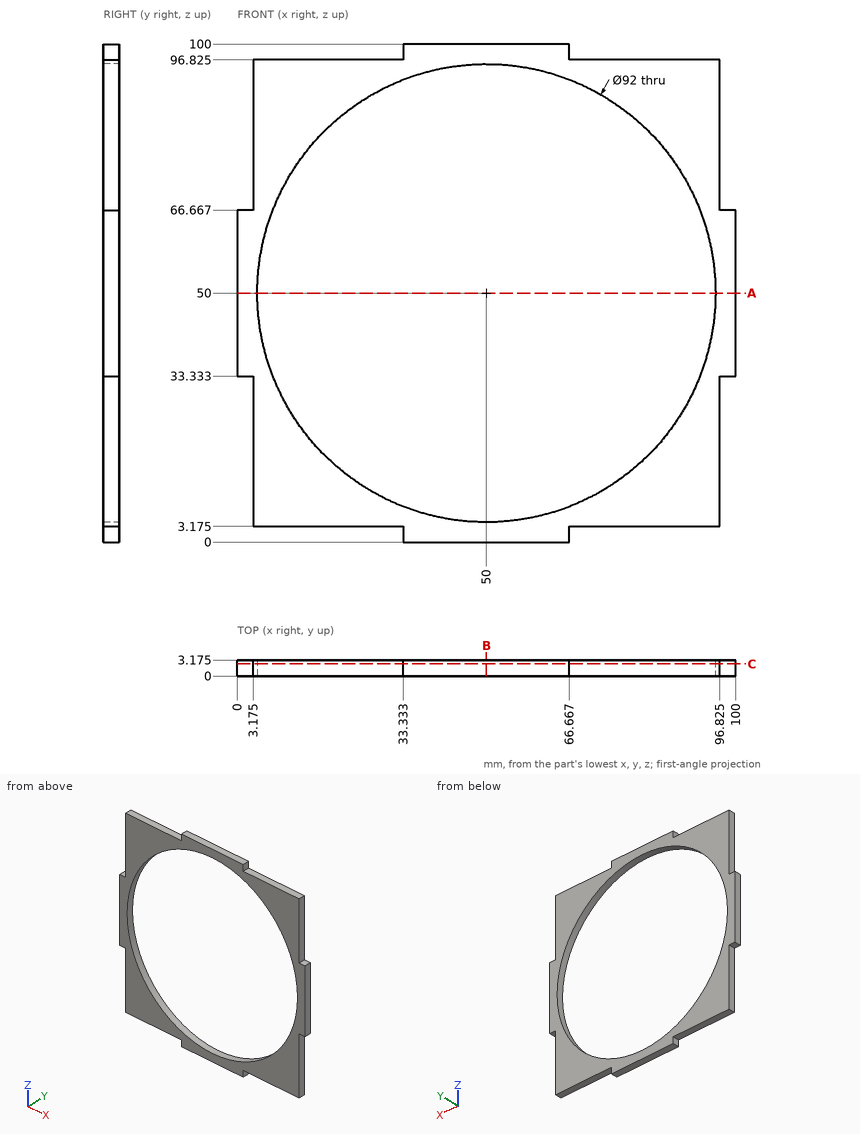
Geometry check sheet. Reference: drawing and pictorial views, mm from the part's lowest x, y, z. Round coordinates to 2 decimals unless told otherwise and drop trailing zeros. Loops run counter-clockwise (first coordinate to the right, second up) from the corner with the lowest first, then second, coordinate; pieces in that order, holes last. Notation, with made-up numbers: M 51,6 L 72,6 A14 cw 72,10 Z; hole C -36,46 d6. An arc over 180 degrees is marked long. Return JSON: item names as keys, results as strings. Group by question number.
(1) Go/stop test with flat-tipped pins: pin 1 (1 mm diameter, centred on y = 1.5, z = 1, fed in from -X); pin 2 (1 mm diameter, centred on y = 1, z = 2, fed in from +X); pin 3 (1 mm diameter, centred on y = 2, z = 21, fed in from -X) (3 decimals). Record where each tip stops, or that it passes through.
(2) Section check A-A, the plane z = 50. Enter the section's corners in (x, y) (1 decimal), and give its area (3 significant figures).
(3) Section check C-C, the plane y = 2.45. Enter the section's corners in (x, z) (1 decimal).
(4) Section check B-B, the plane x = 50. Enter the section's corners in (y, z) (1 decimal), and give its area (3 significant figures).
(5) Scan lines: line 1 along X through (y, z) = (1.9, 50); line 2 along Z through (x, y) = (76.5, 3) (1 decimal). Record each from-to range of solid material in increasing order. Write a range as [from, to].
Data:
{
 "1": {"pin 1": "x = 33.33", "pin 2": "x = 66.67", "pin 3": "x = 3.175"},
 "2": {"outline": "M 0,0 L 4,0 L 4,3.2 L 0,3.2 Z; M 96,0 L 100,0 L 100,3.2 L 96,3.2 Z", "area": "25.4 mm²"},
 "3": {"outline": "M 0,33.3 L 3.2,33.3 L 3.2,3.2 L 33.3,3.2 L 33.3,0 L 66.7,0 L 66.7,3.2 L 96.8,3.2 L 96.8,33.3 L 100,33.3 L 100,66.7 L 96.8,66.7 L 96.8,96.8 L 66.7,96.8 L 66.7,100 L 33.3,100 L 33.3,96.8 L 3.2,96.8 L 3.2,66.7 L 0,66.7 Z; hole C 50,50 d92"},
 "4": {"outline": "M 0,0 L 3.2,0 L 3.2,4 L 0,4 Z; M 0,96 L 3.2,96 L 3.2,100 L 0,100 Z", "area": "25.4 mm²"},
 "5": {"line 1": "[0, 4], [96, 100]", "line 2": "[3.2, 12.4], [87.6, 96.8]"}
}
